from build123d import *

# Parameters (mm, degrees)
SKETCH1_R           = 15
BOSS_EXTRUDE1_DEPTH = 70
SKETCH2_R           = 14
BOSS_EXTRUDE2_DEPTH = 16
SKETCH3_R           = 0.5
SKETCH4_R           = 13
CUT_EXTRUDE1_DEPTH  = 78
SKETCH5_R           = 2
CUT_EXTRUDE2_DEPTH  = 9
SKETCH6_W           = 1
SKETCH6_H           = 0.792029488
BOSS_EXTRUDE3_DEPTH = 75
CIRPATTERN1_COUNT   = 3
SKETCH7_R           = 14
CUT_EXTRUDE3_DEPTH  = 5
SCALE1_SCALE        = 0.655
SKETCH8_R           = 9.17
SKETCH8_R_2         = 8.515
BOSS_EXTRUDE4_DEPTH = 9


with BuildPart() as part:
    # Sketch1 → Boss-Extrude1 (new body)
    with BuildSketch(Plane(origin=(0, 0, 0), x_dir=(1, 0, 0), z_dir=(0, 1, 0))):
        Circle(SKETCH1_R)
    extrude(amount=BOSS_EXTRUDE1_DEPTH)

    # Sketch2 → Boss-Extrude2 (add)
    with BuildSketch(Plane(origin=(0, 70, 0), x_dir=(1, 0, 0), z_dir=(0, 1, 0))):
        Circle(SKETCH2_R)
    extrude(amount=BOSS_EXTRUDE2_DEPTH)

    # Sketch3 → Revolve1 (revolve)
    with BuildSketch(Plane.XY):
        with Locations((-14, 73.5)):
            Circle(SKETCH3_R)
    revolve(axis=Axis((0, 70, 0), (0, 1, 0)))

    # Sketch4 → Cut-Extrude1 (cut)
    with BuildSketch(Plane(origin=(0, 86, 0), x_dir=(1, 0, 0), z_dir=(0, 1, 0))):
        Circle(SKETCH4_R)
    extrude(amount=-CUT_EXTRUDE1_DEPTH, mode=Mode.SUBTRACT)

    # Sketch5 → Cut-Extrude2 (cut, through all)
    with BuildSketch(Plane(origin=(0, 8, 0), x_dir=(1, 0, 0), z_dir=(0, 1, 0))):
        Circle(SKETCH5_R)
    extrude(amount=-CUT_EXTRUDE2_DEPTH, mode=Mode.SUBTRACT)

    # Sketch6 → Boss-Extrude3 (add)
    with BuildSketch(Plane(origin=(0, 8, 0), x_dir=(1, 0, 0), z_dir=(0, 1, 0))):
        with Locations((0, 12.896014744)):
            Rectangle(SKETCH6_W, SKETCH6_H)
    boss_extrude3 = extrude(amount=BOSS_EXTRUDE3_DEPTH)

    # CirPattern1: Boss-Extrude3 ×3 about axis
    cirpattern1_axis = Axis((0, 0, 0), (0, 1, 0))
    for i in range(1, CIRPATTERN1_COUNT):
        add(boss_extrude3.rotate(cirpattern1_axis, i * 360 / CIRPATTERN1_COUNT))

    # Sketch7 → Cut-Extrude3 (cut)
    with BuildSketch(Plane.XZ):
        Circle(SKETCH7_R)
    extrude(amount=-CUT_EXTRUDE3_DEPTH, mode=Mode.SUBTRACT)


with BuildPart() as part_1:
    # Scale1: scaled about (0, 0, 0)
    add(part.part.scale(SCALE1_SCALE))

    # Sketch8 → Boss-Extrude4 (add)
    with BuildSketch(Plane(origin=(0, 56.33, 0), x_dir=(1, 0, 0), z_dir=(0, 1, 0))):
        Circle(SKETCH8_R)
        Circle(SKETCH8_R_2, mode=Mode.SUBTRACT)
    extrude(amount=BOSS_EXTRUDE4_DEPTH)


solid = part_1.part
Verification items for the finished model (mm, model axes). A direction names the side the tool comes from. Coordinates: 2 decimals unless noted, no trailing zeros. Put each result on its own line as item: value. Start each with the question number.
1. Mould release check, pull along Y, two halves, no side actions. Record for faces 4 (the cylindrical face through (-1.99, 46.82, 8.95)), 5 (the flat face through (-3, 0, 9)), 6 (the cylindrical face through (-1.99, 1.61, -8.95)): released by +Y, released by -Y, zero draft, split by the parting line, or undercut.
2. Material ranges on L1, parallel to Z at x = 0, y = 39.5 (1 decimal); L2, parallel to X at y = 62.25, z = 0 (3 decimals), recorded low to high. Write a range as [from, to].
3. Go/stop test with flat-tipped pins: pin 1 Ø10 at (x, z) = (0.5, 0) entering from +Y; pin 2 Ø4 at (x, z) = (0, 0) entering from -Y (3 decimals); pin 3 Ø3 at (x, y) = (3.5, 15) entering from -Z. Record where each tip stops, or that it passes through.
4. Access from +Z, -Z, +X, -X, +Y, -Y to the whole of each face (thin tool, end or side, straight path). Record for faces 1 (the cylindrical face through (-1.99, 56.78, 8.95)), 2 (the flat face through (-3, 45.85, 9)), 3 (the flat face through (0, 3.275, -2)).
Computed:
1. face 4: undercut
1. face 5: released by -Y
1. face 6: zero draft
2. L1: [-9.8, -8.2], [8.5, 9.8]
2. L2: [-9.17, -8.515], [8.515, 9.17]
3. pin 1: y = 5.24
3. pin 2: y = 3.275
3. pin 3: z = -9.62
4. face 1: +Y
4. face 2: none
4. face 3: -Y
